Autodesk Inventor part; units mm, degrees
ref_plane "YZ Plane" through (0, 0, 0) normal (1, 0, 0) x (0, 1, 0)
ref_plane "XZ Plane" through (0, 0, 0) normal (0, 1, 0) x (-1, 0, 0)
ref_plane "XY Plane" through (0, 0, 0) normal (0, 0, 1) x (1, 0, 0)
sketch "Sketch1" plane through (0, 0, 0) normal (0, 0, 1) x (1, 0, 0)
  line L0 (-38.1, 38.1) -> (38.1, 38.1)
  line L1 (38.1, 38.1) -> (38.1, -38.1)
  line L2 (38.1, -38.1) -> (-38.1, -38.1)
  line L3 (-38.1, -38.1) -> (-38.1, 38.1)
  line L4 (-38.1, 38.1) -> (38.1, -38.1) construction
  line L5 (38.1, 38.1) -> (-38.1, -38.1) construction
  point P0 (0, 0)
  dimension "d0" = 76.2
  dimension "d1" = 76.2
extrude "Extrusion1" add sketch "Sketch1" along normal blind 0.7937
sketch "Sketch2" plane through (0, 0, 0.7937) normal (0, 0, 1) x (1, 0, 0)
  line L0 (38.1, 38.1) -> (-38.1, 38.1)
  line L1 (-38.1, 38.1) -> (-38.1, -38.1)
  line L2 (-38.1, -38.1) -> (38.1, -38.1)
  line L3 (38.1, -38.1) -> (38.1, 38.1)
  line L4 (-31.75, 31.75) -> (31.75, 31.75)
  line L5 (31.75, 31.75) -> (31.75, -31.75)
  line L6 (31.75, -31.75) -> (-31.75, -31.75)
  line L7 (-31.75, -31.75) -> (-31.75, 31.75)
  point P0 (0, 0)
  point P1 (0, 31.75)
  point P2 (31.75, 0)
  point P3 (0, -31.75)
  point P4 (-31.75, 0)
  dimension "d7" = 6.35
chamfer "Chamfer1" distance 6.35 angle 45 4 edges at (38.1, 38.1, 0.3969) (-38.1, 38.1, 0.3969) (38.1, -38.1, 0.3969) (-38.1, -38.1, 0.3969)
hole "Hole1" at (-31.75, 31.75, 0.7937) at (0, 31.75, 0.7937) at (31.75, 31.75, 0.7937) at (31.75, 0, 0.7937) at (31.75, -31.75, 0.7937) at (0, -31.75, 0.7937) at (-31.75, -31.75, 0.7937) at (-31.75, 0, 0.7937) direction (0, 0, -1) diameter 3.264 end through all
sketch "Sketch3" plane through (0, 0, 0.7937) normal (0, 0, 1) x (1, 0, 0)
  line L0 (-25.4, -25.4) -> (25.4, -25.4)
  line L1 (25.4, -25.4) -> (25.4, 25.4)
  line L2 (25.4, 25.4) -> (-25.4, 25.4)
  line L3 (-25.4, 25.4) -> (-25.4, -25.4)
  line L4 (-25.4, -25.4) -> (25.4, 25.4) construction
  line L5 (25.4, -25.4) -> (-25.4, 25.4) construction
  point P0 (0, 0)
  dimension "d15" = 50.8
  dimension "d16" = 50.8
extrude "Extrusion2" cut sketch "Sketch3" against normal through all
equation "\"d7\" = backplaneHoleOffsett"
equation "\"frameAcrylicThickness\" = 9.525"
equation "\"internalAcrylicThickness\" = 6.35"
equation "\"height\" = 127"
equation "\"width\" = 127"
equation "\"depth\" = 273.05"
equation "\"mirrorAngle\" = 5deg"
equation "\"detectorWidth\" = 52"
equation "\"detectorHeight\" = 52"
equation "\"mirrorThickness\" = 3.175"
equation "\"fresnelThickness\" = 0.1"
equation "\"focalLength\" = 76.2"
equation "\"ior\" = 1.49"
equation "\"centerThickness\" = 1.524"
equation "\"fresnelAngle\" = 90deg"
equation "\"fresnelEffectiveDiameter\" = 152.4"
equation "\"oRingWidth\" = 1.5875"
equation "\"sensorHolderDepth\" = 19.05"
equation "\"aerogelClearence\" = 3.175"
equation "\"backplanePCBWidth\" = 76.2"
equation "\"backplanePCBHeight\" = 76.2"
equation "\"backplaneHoleOffsett\" = 6.35"
equation "\"backplanePostionOffsett\" = 12.7"
equation "\"moduleSlotClearence\" = 0.79375"
properties part number "backplaneGasket" material "Rubber"
Can you work these out from the model? Positions are in its coordinate system, mm. Coordinates: 2 decimals unless noted, no trailing zeros. Loops run counter-clockwise (first coordinate to the right, second up) from the corner with the lowest first, then second, coordinate; pieces in that order, holes last. Notation, with made-up numbers: (8, 60) -> (59, 60) arc R20 ccw to (59, 94) -> close; hole circle Ø5 at (-15.75, -22.5). An arc over 180 degrees is marked (long way). Put each result on its own line as item: value. Start each with the question number.
Q1. I want a section at C-C (y = 15.5). Write out the boundary of the cut face in (x, z), plus the area to 3 significant figures.
Q2. I want a section at D-D (z = 0.3). Count the separate pieces of the cut face and the enclosed holes in it, plus the area to 3 significant figures.
Q3. Thinking about a two-plate mould opening in X: for faces 1 (the face through (34.97, 34.88, 0.39)), 2 (the face through (-26, 1, 0.794)), 3 (the face through (-33.126, 30.873, 0.391)), which applies, pulls with the +X half, pulls with the -X half, needs draft (parallel to the pull), parting line crosses it, or undercut?
Q4. If I drill on line 1 (Y direction, x = 31.75, z = 0.25); line 2 (X direction, y = 0, z = 0.55), over which ranges is the centre line in solid material (lowest first)? Write a range as [from, to].
Q5. I want a section at A-A (y = 0). Write out the boundary of the cut face in (x, z).
Taken from the geometry:
1. outline: (-38.1, 0) -> (-25.4, 0) -> (-25.4, 0.79) -> (-38.1, 0.79) -> close; (25.4, 0) -> (38.1, 0) -> (38.1, 0.79) -> (25.4, 0.79) -> close
1. area: 20.2 mm2
2. separate pieces: 1
2. enclosed holes: 9
2. area: 3,080 mm2
3. face 1: pulls with the +X half
3. face 2: needs draft
3. face 3: undercut
4. line 1: y = [-38.1, -33.38], [-30.12, -1.63], [1.63, 30.12], [33.38, 38.1]
4. line 2: x = [-38.1, -33.38], [-30.12, -25.4], [25.4, 30.12], [33.38, 38.1]
5. outline: (-38.1, 0) -> (-33.38, 0) -> (-33.38, 0.79) -> (-38.1, 0.79) -> close; (-30.12, 0) -> (-25.4, 0) -> (-25.4, 0.79) -> (-30.12, 0.79) -> close; (25.4, 0) -> (30.12, 0) -> (30.12, 0.79) -> (25.4, 0.79) -> close; (33.38, 0) -> (38.1, 0) -> (38.1, 0.79) -> (33.38, 0.79) -> close
